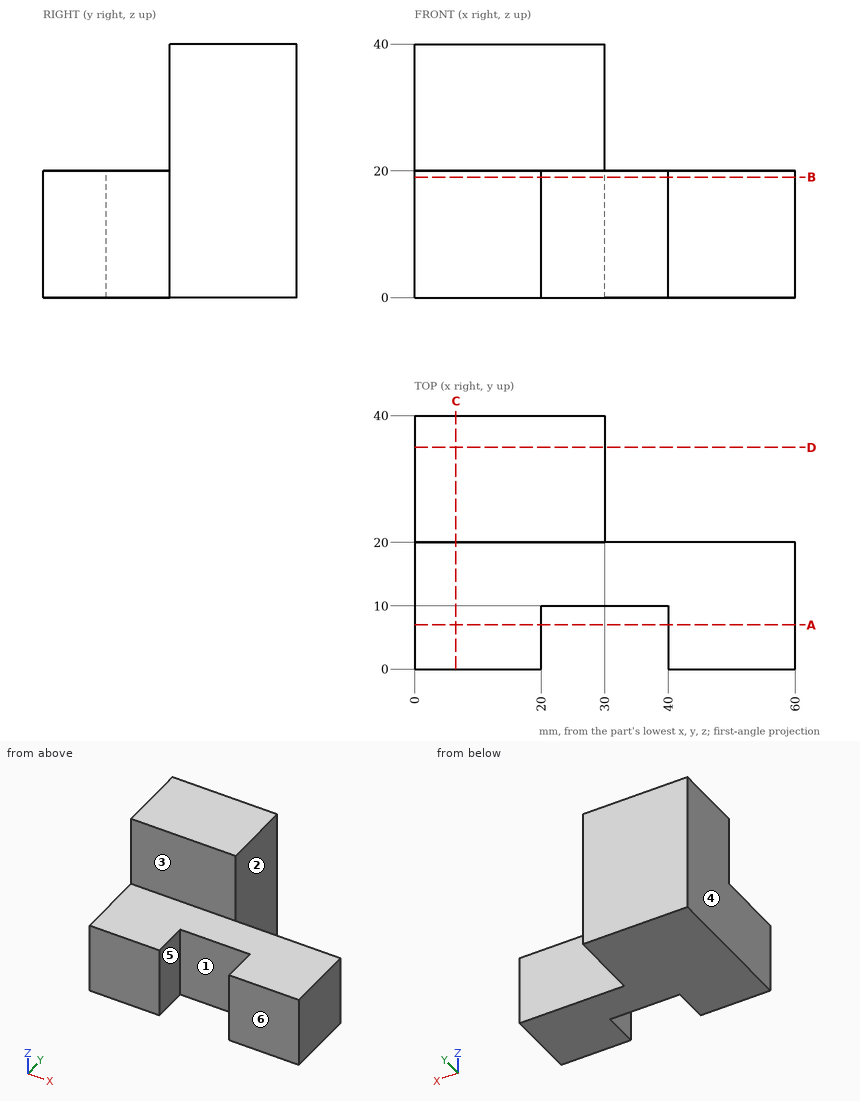
For this review, use the dimensioned drawing (mm, ordinates from the lowest corner) and the shaded views. A direction names the side the tool comes from. Round coordinates to 2 decimals unless told otherwise and drop trailing zeros. Write each loop counter-clockwise with the first axis right and the second up, starting at its lowest first coordinate (ties: lowest second). Pieces come first, ordered by that corner, then holes. Notation, with made-up numbers: (-25, -39) -> (12, -39) arc R25 ccw to (12, -8) -> close; hole circle Ø8 at (62, -36.75). An arc over 180 degrees is marked (long way). Use CSV: the item, a comma, the result in double quotes.
(1) To check wall thickness, follow L1, parallel to X at y = 28, z = 24; L2, parallel to X at y = 4, z = 4.5; L3, parallel to Z at x = 51, y = 3. State the ranges of each line that lie inside material, in increasing order. Write a range as [from, to].
Computed values:
L1,"[0, 30]"
L2,"[0, 20], [40, 60]"
L3,"[0, 20]"
(2) Clearance check with flat-ended pins moving along their axes: P1, Ø2, axis at y = 28.5, z = 12, coming from the +X side; P2, Ø6, axis at x = 28.5, z = 14.5, coming from the -Y side; P3, Ø6, axis at x = 17, z = 34, coming from the -Y side. State where each tip first meets the part, or that it passes through.
Computed values:
P1,"x = 30"
P2,"y = 10"
P3,"y = 20"
(3) For the marked faces 1, 2 and 3, list the 3-axis set-ups (+Z, -Z, +X, -X, +Y, -Y) from which the entire face can be reached by the end or side of a thin tool; tool diameter is ignored.
Computed values:
face 1,"+Z, -Z, -Y"
face 2,"+Z, -Z, +X, +Y"
face 3,"+Z, +X, -X, -Y"
(4) Consider section C-C, the plane x = 6.5. Give the boundary of the cut face in (y, z).
Computed values:
outline,"(0, 0) -> (40, 0) -> (40, 40) -> (20, 40) -> (20, 20) -> (0, 20) -> close"
(5) Consider section B-B, the plane z = 19. Give the boundary of the cut face in (x, y).
Computed values:
outline,"(0, 0) -> (20, 0) -> (20, 10) -> (40, 10) -> (40, 0) -> (60, 0) -> (60, 20) -> (30, 20) -> (30, 40) -> (0, 40) -> close"
(6) Consider section A-A, the plane y = 7. Give the boundary of the cut face in (x, z).
Computed values:
outline,"(0, 0) -> (20, 0) -> (20, 20) -> (0, 20) -> close; (40, 0) -> (60, 0) -> (60, 20) -> (40, 20) -> close"
(7) Draft analysis for pull direction X (two halves, no side actions). For the marked faces 4, 5 and 6, state which applies: +X half, -X half, draft (parallel to the pull), parting line (faces both ways), or undercut.
Computed values:
face 4,"-X half"
face 5,"undercut"
face 6,"draft"
(8) Consider section D-D, the plane y = 35. Give the boundary of the cut face in (x, z).
Computed values:
outline,"(0, 0) -> (30, 0) -> (30, 40) -> (0, 40) -> close"
